Geometry: final body of the model. Coordinates: model frame, mm. A direction names the side the tool comes from. Round coordinates to 2 decimals unless told otherwise and drop trailing zeros. Order: outer loops, then holes, each group sorted by start corner. A loop starts at its lowest first (then second) coordinate and runs counter-clockwise, first axis right, second up. Notation, with made-up numbers: M -28.75,16.5 L 13.25,16.5 A9 cw 13.25,30.5 Z; hole C 59,3.25 d10. An arc over 180 degrees is marked long. Put each result on its own line as item: value. Start each with the question number.
1) Section B-B, the plane y = 1.3. Return loops of the section in (x, z).
2) Section A-A, the plane x = -2.25. Return loops of the section in (y, z), then the cut area to 4 significant figures.
3) Access query for faces 1 (the flat face through (0, 4.75, 4)), 2 (the flat face through (0, 6, 0)), 3 (the flat face through (0, 2.25, 4)), 4 (the flat face through (-2.95, 3, 4)), 5 (the flat face through (2.95, 3, 4)). Directions: +Z, -Z, +X, -X, +Y, -Y. A direction counts if a zero-diameter tool reaches every point of the face in a straight line with its end or side. Return the directions, or none.
4) Section C-C, the plane x = -5.25. Return loops of the section in (y, z), then the cut area to 3 significant figures.
5) Material intervals for probe 1 along Z at (x, y) = (-6, 1.55); probe 2 along X at (y, z) = (3.1, 4.5); probe 3 along Y at (x, z) = (-2.5, 3), sorted ascending. Write a range as [from, to].
6) First-contact query: P1, Ø2, axis at y = 3, z = 4, coming from the -X side; P2, Ø0.8, axis at y = 4, z = 4, coming from the +X side; P3, Ø0.8, axis at x = -1, z = 4.5, coming from the -Y side. Flat tips, straight axial feed; report the tip coordinate or a pass-through.
from build123d import *

# Parameters (mm, degrees)
SKETCH1_W           = 13
SKETCH1_H           = 5.6
BOSS_EXTRUDE1_DEPTH = 6
SKETCH2_W           = 5.9
SKETCH2_H           = 2.5
BOSS_EXTRUDE2_DEPTH = 3
CHAMFER1_SIZE       = 0.5


with BuildPart() as part:
    # Sketch1 → Boss-Extrude1 (new body)
    with BuildSketch(Plane(origin=(0, 0, 0), x_dir=(1, 0, 0), z_dir=(0, 1, 0))):
        Rectangle(SKETCH1_W, SKETCH1_H)
    extrude(amount=BOSS_EXTRUDE1_DEPTH)

    # Sketch2 → Boss-Extrude2 (add)
    with BuildSketch(Plane.XY.offset(2.8)):
        with Locations((0, 3.5)):
            Rectangle(SKETCH2_W, SKETCH2_H)
    extrude(amount=BOSS_EXTRUDE2_DEPTH)

    # Chamfer1
    chamfer1_edges = [part.edges().sort_by_distance(p)[0] for p in [
        (2.95, 3.5, 5.8),
        (0, 4.75, 5.8),
        (-2.95, 3.5, 5.8),
        (0, 2.25, 5.8),
    ]]
    chamfer(chamfer1_edges, length=CHAMFER1_SIZE)


solid = part.part
Result sheet:
1. outline: M -6.5,-2.8 L 6.5,-2.8 L 6.5,2.8 L -6.5,2.8 Z
2. outline: M 0,-2.8 L 6,-2.8 L 6,2.8 L 4.75,2.8 L 4.75,5.3 L 4.25,5.8 L 2.75,5.8 L 2.25,5.3 L 2.25,2.8 L 0,2.8 Z
2. area: 40.85 mm2
3. face 1: +Z, +X, -X, +Y
3. face 2: +Z, -Z, +X, -X, +Y
3. face 3: +Z, +X, -X, -Y
3. face 4: +Z, -X, +Y, -Y
3. face 5: +Z, +X, +Y, -Y
4. outline: M 0,-2.8 L 6,-2.8 L 6,2.8 L 0,2.8 Z
4. area: 33.6 mm2
5. probe 1: z = [-2.8, 2.8]
5. probe 2: x = [-2.95, 2.95]
5. probe 3: y = [2.25, 4.75]
6. P1: stops at x = -2.95
6. P2: stops at x = 2.95
6. P3: stops at y = 2.25
